The model under review builds one solid part; all positions refer to its coordinate system, in mm. A direction names the side the tool comes from. Give positions to 0.01 mm unless a question says otherwise; leave off trailing zeros. Use CSV: the item, a comma, the result in double quotes. Start each with the question number.
```python
from build123d import *

# Parameters (mm, degrees)
SKETCH040_R      = 1.6
SKETCH040_R_2    = 12.5
SKETCH040_R_3    = 3
EXTRUDE004_DEPTH = 10


with BuildPart() as extrude004:
    # Sketch040 → Extrude004 (new body)
    with BuildSketch(Plane.XY.offset(-9.9)):
        with Locations((0, 15)):
            Circle(SKETCH040_R)
        with Locations((0, -15)):
            Circle(SKETCH040_R)
        with Locations((-15, 0)):
            Circle(SKETCH040_R)
        with Locations((15, 0)):
            Circle(SKETCH040_R)
        Circle(SKETCH040_R_2)
        with Locations((15.556349, 15.556349)):
            Circle(SKETCH040_R_3)
    extrude(amount=-EXTRUDE004_DEPTH)


with BuildPart() as cut:
    # Sketch039 → Revolve (revolve)
    with BuildSketch(Plane.XZ):
        Polygon((41, -6.5), (41, -3), (43.3, -3), (43.3, -4.6), (45.3, -4.6), (45.3, -5.4), (39.2, -11.5), (0, -11.5), (0, -9.9), (37.6, -9.9), align=None)
    revolve(axis=Axis((0, 0, 0), (0, 0, 1)))

    # Cut: cut Extrude004
    add(extrude004.part, mode=Mode.SUBTRACT)


solid = cut.part
```
1. Mouldability with a two-part tool opening along X and no side actions: class faces 3 (the face through (-16.6, 0.07, -10.69)), 4 (the face through (-5.142, 39.16, -11.204)), 5 (the face through (-37, -23, -4.6)) as pulls with the +X half, pulls with the -X half, needs draft (parallel to the pull), parting line crosses it, or undercut.
2. To check wall thickness, follow L1, parallel to Y at x = 0, z = -4.35; L2, parallel to Y at x = 0, z = -10.95; L3, parallel to Z at x = -22, y = 14. State the ranges of each line that lie inside material, in increasing order. Write a range as [from, to].
3. Tool access review of faces 1 (the face through (-0.208, -13.414, -10.689)), 2 (the face through (-9, -40, -5)): name each direction out of +Z, -Z, +X, -X, +Y, -Y from which nothing blocks a thin tool from reaching the whole face with its end or side.
4. Consider section A-A (x = 15). State how many separate pieces and enclosed holes the cut face has, and give its area (3 significant figures).
5. Clearance check with flat-ended pins moving along their axes: pin 1 (3.5 mm diameter, centred on x = 0, y = -15, fed in from +Z); pin 2 (5 mm diameter, centred on x = 15.56, y = 15.56, fed in from +Z); pin 3 (12 mm diameter, centred on x = 16.5, y = 30, fed in from +Z). State where each tip first meets the part, or that it passes through.
Answers follow:
1,face 3,"undercut"
1,face 4,"parting line crosses it"
1,face 5,"needs draft"
2,L1,"y = [-43.3, -41], [41, 43.3]"
2,L2,"y = [-39.75, -16.6], [-13.4, -12.5], [12.5, 13.4], [16.6, 39.75]"
2,L3,"z = [-11.5, -9.9]"
3,face 1,"+Z, -Z"
3,face 2,"+Z"
4,separate pieces,"3"
4,enclosed holes,"0"
4,area,"152 mm^2"
5,pin 1,"stops at z = -9.9"
5,pin 2,"passes through"
5,pin 3,"stops at z = -7.26"
